Design review of the part built by this model. Coordinates are the model's own, in mm. A direction names the side the tool comes from. Round coordinates to 2 decimals unless told otherwise and drop trailing zeros. Write each loop counter-clockwise with the first axis right and the second up, starting at its lowest first coordinate (ties: lowest second). Pieces come first, ordered by that corner, then holes. Notation, with made-up numbers: (42, 37.25) -> (53, 37.25) arc R26 ccw to (53, 65.25) -> close; hole circle Ø4 at (69.25, 37.5). An arc over 180 degrees is marked (long way). One line per question, with ' | ' between items. Start each with the question number.
1) For probe 1 along Z at (x, y) = (0, -4); probe 2 along Z at (x, y) = (-4, -8); probe 3 along Z at (x, y) = (-113, -2.5), list the stretches that pass through material, from the lowest coordinate up.
2) Insertion check: pin 1 Ø3 at (x, y) = (-113, -6) entering from -Z; pin 2 Ø3 at (y, z) = (-5, 91.5) entering from -X; pin 3 Ø5 at (y, z) = (-4.5, -78.5) entering from -X; pin 4 Ø5 at (x, y) = (-104, -4) entering from +Z. Each pin has a flat end and moves straight along its axis. Give the tip position at first contact, or say it passes through.
3) Consider section A-A (x = -113). Give the boundary of the cut face in (y, z).
4) For faces 1 (the flat face through (25, -5, 122)), 2 (the flat face through (0, -5, -102)), 3 (the flat face through (-75, -5, -159)), 4 (the flat face through (-25, -5, 123)), 5 (the flat face through (-115, -5, -80)), list the 3-axis set-ups (+Z, -Z, +X, -X, +Y, -Y) from which the entire face can be reached by the end or side of a thin tool; tool diameter is ignored.
5) Consider section B-B (z = 0). Give the boundary of the cut face in (x, y), then the cut area to 3 significant figures.
6) Mouldability with a two-part tool opening along Z and no side actions: class faces 6 (the flat face through (25, -5, -131)), 7 (the cylindrical face through (-91.137, -5.07, 12.573)), 8 (the flat face through (-26, -5, -167.5)) as +Z half, -Z half, draft (parallel to the pull), parting line (faces both ways), or undercut.
7) Consider section D-D (x = 0). Give the boundary of the cut face in (y, z).
8) Consider section C-C (y = -5.25). Give the boundary of the cut face in (x, z), then the cut area to 3 significant figures.
```python
from build123d import *

# Parameters (mm, degrees)
F1_DEPTH = 10
F2_R     = 98
F2_R_2   = 92
F3_DEPTH = 10
F4_W     = 100
F4_H     = 10
F5_DEPTH = 17.5
F6_W     = 20
F6_H     = 20
F6_H_2   = 30
F6_R     = 3.5
F7_DEPTH = 10


with BuildPart() as f1:
    # F0 (on Front) → F1 (new body)
    with BuildSketch(Plane.XZ):
        Polygon((25, 150), (-25, 150), (-25, -80), (-175, -80), (-175, -150), (25, -150), align=None)
    extrude(amount=F1_DEPTH)

    # F2 (on face) → F3 (join)
    with BuildSketch(Plane.XZ.offset(10)):
        Circle(F2_R)
        Circle(F2_R_2, mode=Mode.SUBTRACT)
    extrude(amount=-F3_DEPTH)

    # F4 (on face) → F5 (join)
    with BuildSketch(Plane(origin=(0, 0, -150), x_dir=(1, 0, 0), z_dir=(0, 0, -1))):
        with Locations((-25, 5)):
            Rectangle(F4_W, F4_H)
    extrude(amount=F5_DEPTH)

    # F6 (on face) → F7 (cut)
    with BuildSketch(Plane.XZ.offset(10)):
        with Locations((0, -92)):
            Rectangle(F6_W, F6_H)
        with Locations((0, 95)):
            Rectangle(F6_W, F6_H_2)
        Circle(F6_R)
        with Locations((-113, -108)):
            Circle(F6_R)
    extrude(amount=-F7_DEPTH, mode=Mode.SUBTRACT)


solid = f1.part
```
From the geometry:
1) probe 1: z = -167.5 to -102, -82 to -3.5, 3.5 to 80, 110 to 150 | probe 2: z = -167.5 to -102, -82 to 80, 110 to 150 | probe 3: z = -150 to -111.5, -104.5 to -80
2) pin 1: stops at z = -150 | pin 2: stops at x = -38.78 | pin 3: stops at x = -175 | pin 4: stops at z = -80
3) outline: (-10, -150) -> (0, -150) -> (0, -111.5) -> (-10, -111.5) -> close; (-10, -104.5) -> (0, -104.5) -> (0, -80) -> (-10, -80) -> close
4) face 1: +Z, +X, +Y, -Y | face 2: +Y, -Y | face 3: -Z, -X, +Y, -Y | face 4: +Z, -X, +Y, -Y | face 5: -X, +Y, -Y
5) outline: (-98, -10) -> (-92, -10) -> (-92, 0) -> (-98, 0) -> close; (-25, -10) -> (-3.5, -10) -> (-3.5, 0) -> (-25, 0) -> close; (3.5, -10) -> (25, -10) -> (25, 0) -> (3.5, 0) -> close; (92, -10) -> (98, -10) -> (98, 0) -> (92, 0) -> close | area: 550 mm2
6) face 6: draft | face 7: undercut | face 8: -Z half
7) outline: (-10, -167.5) -> (0, -167.5) -> (0, -102) -> (-10, -102) -> close; (-10, -82) -> (0, -82) -> (0, -3.5) -> (-10, -3.5) -> close; (-10, 3.5) -> (0, 3.5) -> (0, 80) -> (-10, 80) -> close; (-10, 110) -> (0, 110) -> (0, 150) -> (-10, 150) -> close
8) outline: (-175, -150) -> (-75, -150) -> (-75, -167.5) -> (25, -167.5) -> (25, -94.76) arc R98 ccw to (25, 94.76) -> (25, 150) -> (-25, 150) -> (-25, 94.76) arc R98 ccw to (-56.6, -80) -> (-175, -80) -> close; hole circle Ø7 at (-113, -108); hole (-45.43, -80) -> (-25, -80) -> (-25, 88.54) arc R92 ccw to start; hole (-10, -102) -> (10, -102) -> (10, -82) -> (-10, -82) -> close; hole (-10, 80) -> (10, 80) -> (10, 110) -> (-10, 110) -> close; hole circle Ø7 at (0, 0); hole (25, -88.54) arc R92 ccw to (25, 88.54) -> close | area: 29,000 mm2
